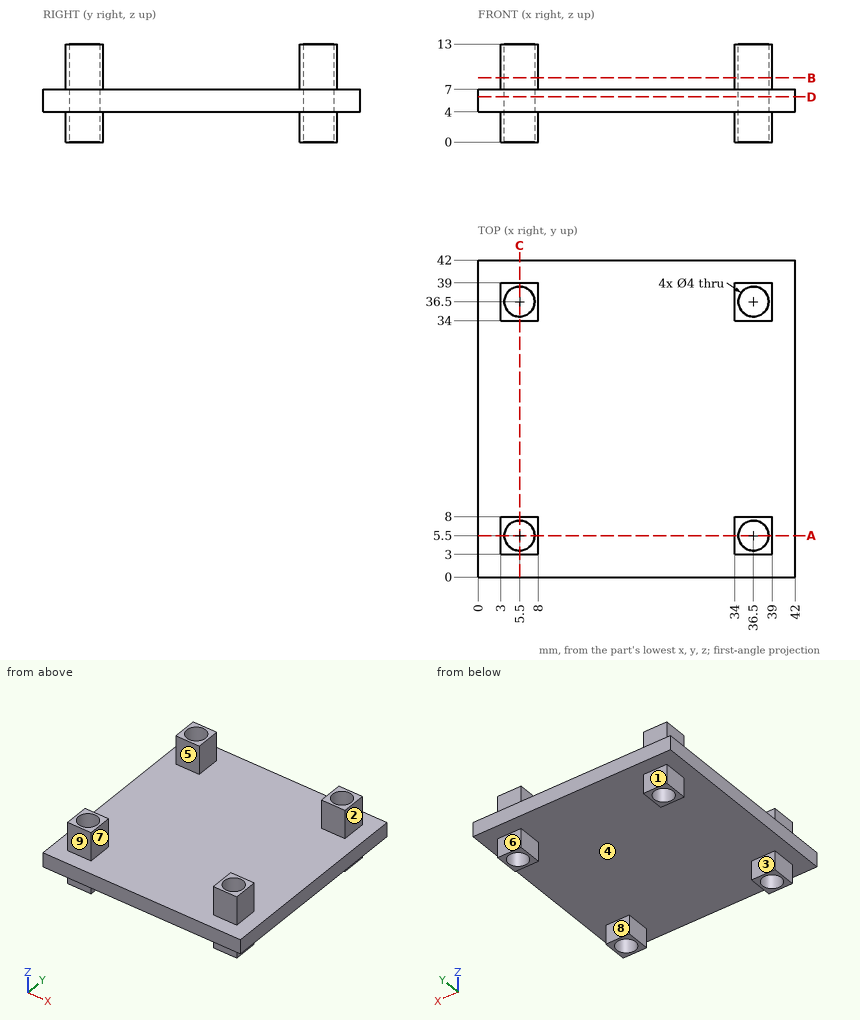
Job drawing, mm, ordinate dimensions from the low corner. One solid piece. A direction names the side the tool comes from. Give positions to 0.01 mm unless a question says otherwise; leave off trailing zeros. Loops run counter-clockwise (first coordinate to the right, second up) from the corner with the lowest first, then second, coordinate; pieces in that order, holes last. Notation, with made-up numbers: (52.5, 31) -> (68.5, 31) arc R23 ccw to (68.5, 67) -> close; hole circle Ø7 at (53, 4). An arc over 180 degrees is marked (long way). Write each question's results on one line, items separated by ' | '.
(1) Cut at A-A on y = 5.5. List the corners of the cut face in (x, z), and give its area (3 significant figures).
Geometry results:
outline: (0, 4) -> (3, 4) -> (3, 0) -> (3.5, 0) -> (3.5, 13) -> (3, 13) -> (3, 7) -> (0, 7) -> close; (7.5, 0) -> (8, 0) -> (8, 4) -> (34, 4) -> (34, 0) -> (34.5, 0) -> (34.5, 13) -> (34, 13) -> (34, 7) -> (8, 7) -> (8, 13) -> (7.5, 13) -> close; (38.5, 0) -> (39, 0) -> (39, 4) -> (42, 4) -> (42, 7) -> (39, 7) -> (39, 13) -> (38.5, 13) -> close | area: 122 mm²
(2) Cut at D-D on z = 6. List the corners of the cut face in (x, y).
Geometry results:
outline: (0, 0) -> (42, 0) -> (42, 42) -> (0, 42) -> close; hole circle Ø4 at (5.5, 5.5); hole circle Ø4 at (5.5, 36.5); hole circle Ø4 at (36.5, 5.5); hole circle Ø4 at (36.5, 36.5)
(3) Probe line 1 along X through (y, z) = (36.5, 10); line 2 along Y through (x, z) = (36.5, 4.25). List the from-to ranges inside material, lowest first.
Geometry results:
line 1: x = 3 to 3.5, 7.5 to 8, 34 to 34.5, 38.5 to 39 | line 2: y = 0 to 3.5, 7.5 to 34.5, 38.5 to 42
(4) Tool access for the marked faces 5, 6, 7, 8 and 9: list every direction of +Z, -Z, +X, -X, +Y, -Y with a clear straight run to the whole face (end or side of a thin tool).
Geometry results:
face 5: +Z, +X, -X | face 6: -Z, +X, -X, +Y | face 7: +Z, +Y, -Y | face 8: -Z, +X, -X | face 9: +Z, +X, -X, -Y
(5) Pull direction Y, two halves, no side cores. Call the marked faces 1, 2, 3 and 4: released by +Y, released by -Y, zero draft, split by the parting line, or undercut.
Geometry results:
face 1: released by +Y | face 2: zero draft | face 3: undercut | face 4: undercut
(6) Flat gauge pins, fed straight in: pin 1 Ø3 at (x, y) = (17, 14) entering from +Z; pin 2 Ø1.2 at (y, z) = (36.5, 1.5) entering from -X; pin 3 Ø4.5 at (x, z) = (37, 1.5) entering from +Y; pin 4 Ø4.5 at (y, z) = (6.5, 2.5) entering from -X. Where does each tip first touch, or does it go through?
Geometry results:
pin 1: stops at z = 7 | pin 2: stops at x = 3 | pin 3: stops at y = 39 | pin 4: stops at x = 0
(7) Cut at B-B on z = 8.5. List the corners of the cut face in (x, y), and give its area (3 significant figures).
Geometry results:
outline: (3, 3) -> (8, 3) -> (8, 8) -> (3, 8) -> close; (3, 34) -> (8, 34) -> (8, 39) -> (3, 39) -> close; (34, 3) -> (39, 3) -> (39, 8) -> (34, 8) -> close; (34, 34) -> (39, 34) -> (39, 39) -> (34, 39) -> close; hole circle Ø4 at (5.5, 5.5); hole circle Ø4 at (5.5, 36.5); hole circle Ø4 at (36.5, 5.5); hole circle Ø4 at (36.5, 36.5) | area: 49.7 mm²
